from build123d import *

# Parameters (mm, degrees)
SKETCH1_R               = 3.8
SKETCH1_R_2             = 1.75
SKETCH1_R_3             = 2.2
BOSS_EXTRUDE1_DEPTH     = 4
BOSS_EXTRUDE2_DEPTH     = 70
CUT_EXTRUDE1_DEPTH      = 10
CUT_EXTRUDE1_DEPTH_BACK = 17
SKETCH6_W               = 5
SKETCH6_H               = 3
BOSS_EXTRUDE4_DEPTH     = 5
SKETCH7_R               = 1.75
CUT_EXTRUDE2_DEPTH      = 35


with BuildPart() as part:
    # Sketch1 → Boss-Extrude1 (new body)
    with BuildSketch(Plane(origin=(0, 0, 0), x_dir=(1, 0, 0), z_dir=(0, 1, 0))):
        with BuildLine():
            Line((-91.885, 12.5), (91.885, 12.5))
            ThreePointArc((91.885, 12.5), (104.385, 0), (91.885, -12.5))
            Line((91.885, -12.5), (-91.885, -12.5))
            ThreePointArc((-91.885, -12.5), (-104.385, 0), (-91.885, 12.5))
        make_face()
        with Locations(Location((71.5, 0, 0), (0, 0, 270))):
            Circle(SKETCH1_R, mode=Mode.SUBTRACT)
        with Locations(Location((-91.885, 8.75, 0), (0, 0, 270))):
            Circle(SKETCH1_R_2, mode=Mode.SUBTRACT)
        with Locations(Location((-91.885, -8.75, 0), (0, 0, 270))):
            Circle(SKETCH1_R_2, mode=Mode.SUBTRACT)
        with Locations(Location((-83.385, 0, 0), (0, 0, 270))):
            Circle(SKETCH1_R, mode=Mode.SUBTRACT)
        with Locations(Location((-71.885, 0, 0), (0, 0, 270))):
            Circle(SKETCH1_R_3, mode=Mode.SUBTRACT)
        with Locations(Location((60, 0, 0), (0, 0, 270))):
            Circle(SKETCH1_R_3, mode=Mode.SUBTRACT)
        with Locations(Location((80, 8.75, 0), (0, 0, 270))):
            Circle(SKETCH1_R_2, mode=Mode.SUBTRACT)
        with Locations(Location((80, -8.75, 0), (0, 0, 270))):
            Circle(SKETCH1_R_2, mode=Mode.SUBTRACT)
    extrude(amount=BOSS_EXTRUDE1_DEPTH)

    # Sketch2 → Boss-Extrude2 (add)
    with BuildSketch(Plane(origin=(0, 4, 0), x_dir=(1, 0, 0), z_dir=(0, 1, 0))):
        with BuildLine():
            Line((95.073755841, -12.086431905), (95.073755841, 12.086431905))
            ThreePointArc((95.073755841, 12.086431905), (104.495591505, 0), (95.073755841, -12.086431905))
        make_face()
    extrude(amount=BOSS_EXTRUDE2_DEPTH)

    # Sketch5 → Cut-Extrude1 (cut, two sides: drawn at the far end of the back side and taken through both)
    with BuildSketch(Plane.ZY.offset(-95.073755841).offset(-CUT_EXTRUDE1_DEPTH_BACK)):
        with BuildLine():
            Line((-1.75, 39), (-1.75, 69))
            ThreePointArc((-1.75, 69), (0, 70.75), (1.75, 69))
            Line((1.75, 69), (1.75, 39))
            ThreePointArc((1.75, 39), (0, 37.25), (-1.75, 39))
        make_face()
    extrude(amount=CUT_EXTRUDE1_DEPTH + CUT_EXTRUDE1_DEPTH_BACK, mode=Mode.SUBTRACT)

    # Sketch6 → Boss-Extrude4 (add)
    with BuildSketch(Plane(origin=(0, 4, 0), x_dir=(1, 0, 0), z_dir=(0, 1, 0))):
        with Locations((89.385, -11)):
            Rectangle(SKETCH6_W, SKETCH6_H)
        with Locations((29.385, -11)):
            Rectangle(SKETCH6_W, SKETCH6_H)
        with Locations((11.885, -11)):
            Rectangle(SKETCH6_W, SKETCH6_H)
        with Locations((-5.615, -11)):
            Rectangle(SKETCH6_W, SKETCH6_H)
        with Locations((-23.115, -11)):
            Rectangle(SKETCH6_W, SKETCH6_H)
        with Locations((-40.615, -11)):
            Rectangle(SKETCH6_W, SKETCH6_H)
        with Locations((89.385, 11)):
            Rectangle(SKETCH6_W, SKETCH6_H)
        with Locations((29.385, 11)):
            Rectangle(SKETCH6_W, SKETCH6_H)
        with Locations((11.885, 11)):
            Rectangle(SKETCH6_W, SKETCH6_H)
        with Locations((-5.615, 11)):
            Rectangle(SKETCH6_W, SKETCH6_H)
        with Locations((-23.115, 11)):
            Rectangle(SKETCH6_W, SKETCH6_H)
        with Locations((-40.615, 11)):
            Rectangle(SKETCH6_W, SKETCH6_H)
    extrude(amount=BOSS_EXTRUDE4_DEPTH)

    # Sketch7 → Cut-Extrude2 (cut)
    with BuildSketch(Plane.XY.offset(12.5)):
        with Locations((89.385, 6.5)):
            Circle(SKETCH7_R)
        with Locations((29.385, 6.5)):
            Circle(SKETCH7_R)
        with Locations((11.885, 6.5)):
            Circle(SKETCH7_R)
        with Locations((-5.615, 6.5)):
            Circle(SKETCH7_R)
        with Locations((-23.115, 6.5)):
            Circle(SKETCH7_R)
        with Locations((-40.615, 6.5)):
            Circle(SKETCH7_R)
    extrude(amount=-CUT_EXTRUDE2_DEPTH, mode=Mode.SUBTRACT)


solid = part.part
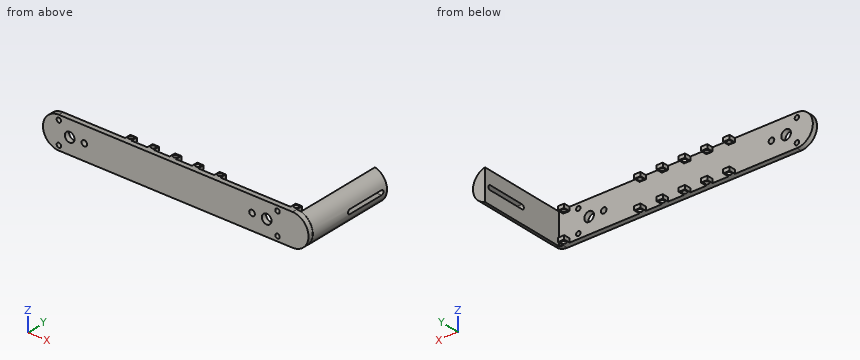
Source: CAD feature listing. Evaluate the final solid. Frame: model axes, mm. Give positions to 0.01 mm unless a question says otherwise; leave off trailing zeros. Write each loop counter-clockwise with the first axis right and the second up, starting at its lowest first coordinate (ties: lowest second). Pieces come first, ordered by that corner, then holes. Notation, with made-up numbers: M 51.25,53 L 98.25,53 A23 cw 98.25,67 Z; hole C 62,-28.5 d2. An arc over 180 degrees is marked long. Return JSON: item names as keys, results as strings. Group by question number.
1) Ray query, L1, parallel to Z at x = 80, y = 3.1; L2, parallel to X at y = 61, z = 2; L3, parallel to Y at x = -3, z = 5.5. Return the intervals inside material, ascending.
2) Cut plane B-B, the plane x = 3.5. Output: boundary loops of the cut face in (y, z).
3) Cut plane C-C, the plane y = 23.5. Output: boundary loops of the cut face in (x, z), then the cut area to 3 significant figures.
4) First-contact query: pin 1 Ø0.9 at (y, z) = (6.5, -11) entering from -X (3 decimals); pin 2 Ø2.5 at (x, z) = (12.5, 11.5) entering from +Y; pin 3 Ø3 at (y, z) = (49.5, -2) entering from -X; pin 4 Ø3 at (x, y) = (-40.615, 6.5) entering from +Z. Flat tips, straight axial feed; report the tip coordinate or a pass-through.
5) Cut plane A-A, the plane y = 61. Output: boundary loops of the cut face in (x, z), then the cut area to 3 significant figures.
Data:
{
 "1": {"L1": "z = -12.5 to -10.5, -7 to 7, 10.5 to 12.5", "L2": "x = 95.07 to 104.33", "L3": "y = 0 to 4"},
 "2": {"outline": "M 0,-12.5 L 4,-12.5 L 4,12.5 L 0,12.5 Z"},
 "3": {"outline": "M 95.07,-12.09 A12.46 ccw 95.07,12.09 Z", "area": "169 mm²"},
 "4": {"pin 1": "stops at x = -43.115", "pin 2": "stops at y = 9", "pin 3": "stops at x = 95.07", "pin 4": "passes through"},
 "5": {"outline": "M 95.07,-12.09 A12.46 ccw 104.37,-1.75 L 95.07,-1.75 Z; M 95.07,1.75 L 104.37,1.75 A12.46 ccw 95.07,12.09 Z", "area": "136 mm²"}
}
